Input: dimensioned drawing with shaded views. Units: mm. Origin: part minimum x, y, z. A direction names the side the tool comes from. Round coordinates to 2 decimals unless told otherwise and drop trailing zeros. Loops run counter-clockwise (first coordinate to the right, second up) from the corner with the lowest first, then second, coordinate; pieces in that order, holes last. Notation, with made-up numbers: M 21.25,73.25 L 72.25,73.25 A10 ccw 72.25,83.25 Z; hole C 29.5,-24 d9. An arc over 180 degrees is marked long. Put each result on its own line as item: value. Start each with the question number.
1) Line query: probe 1 along Y at (x, z) = (21.5, 1.25) (1 decimal); probe 2 along Z at (x, y) = (41, 19.5) (1 decimal). Output: solid intervals per line, ascending.
2) Section C-C on y = 17. Output: boundary loops of the cut face in (x, z) (1 decimal), plus the area to 3 significant figures.
3) Reachability of the marked faces 1 and 2 from +Z, -Z, +X, -X, +Y, -Y: full face, straight path, thin tool, end or side. Return the list, or none.
4) Draft query along X for the marked faces 3, 4 and 5. Return one class per face: +X half, -X half, draft (parallel to the pull), parting line (faces both ways), or undercut.
5) Pin query (flat end, axial travel): pin 1 (1.5 mm diameter, centred on x = 9.5, y = 5.5, fed in from +Z) (1 decimal); pin 2 (2 mm diameter, centred on x = 32.5, z = 2, fed in from -Y); pin 3 (2 mm diameter, centred on x = 21.43, z = 6.35, fed in from +Y). Return the tip coordinate at first contact, or that it passes through.
6) Section A-A on x = 22. Output: boundary loops of the cut face in (y, z) (1 decimal).
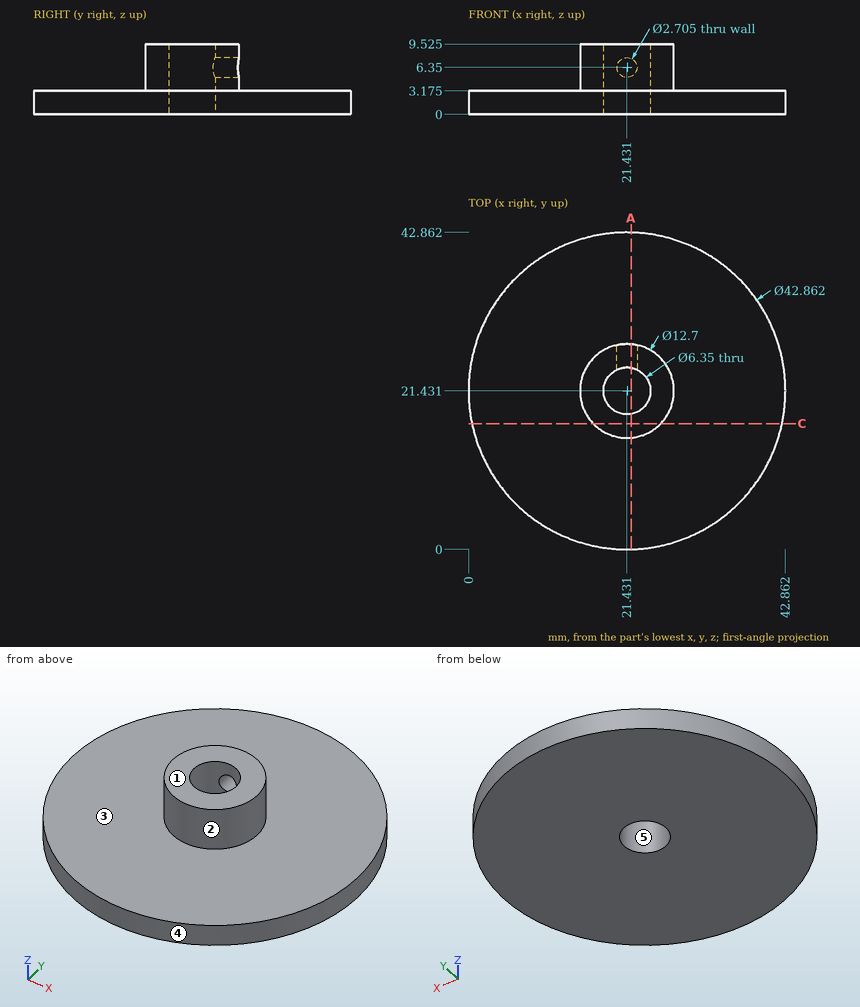
Geometry results:
1. probe 1: y = 0 to 18.3, 24.6 to 42.9
1. probe 2: z = 0 to 3.2
2. outline: M 0.5,0 L 42.4,0 L 42.4,3.2 L 26,3.2 L 26,9.5 L 16.9,9.5 L 16.9,3.2 L 0.5,3.2 Z
2. area: 191 mm²
3. face 1: +Z, +X, -X, +Y, -Y
3. face 2: +Z
4. face 3: draft
4. face 4: parting line
4. face 5: undercut
5. pin 1: stops at z = 3.2
5. pin 2: stops at y = 2.51
5. pin 3: stops at y = 18.42
6. outline: M 0,0 L 18.3,0 L 18.3,9.5 L 15.1,9.5 L 15.1,3.2 L 0,3.2 Z; M 24.6,0 L 42.9,0 L 42.9,3.2 L 27.8,3.2 L 27.8,5.1 L 24.6,5.1 Z; M 24.6,7.6 L 27.8,7.6 L 27.8,9.5 L 24.6,9.5 Z
